```python
from build123d import *

# Parameters (mm, degrees)
SKETCH_1_R      = 2
SKETCH_1_R_2    = 2.08
SKETCH_1_R_3    = 8.75
SKETCH_1_R_4    = 2.2
EXTRUDE_2_DEPTH = 2


with BuildPart() as part:
    # 草图1 → 凸台-拉伸2 (new body)
    with BuildSketch(Plane.XY):
        with BuildLine():
            Line((41.5, 13.75), (41.5, 17))
            Line((41.5, 17), (37, 17))
            Line((37, 17), (37, 20))
            Line((37, 20), (30, 20))
            Line((30, 20), (30, 17))
            Line((30, 17), (25.488968202, 17))
            ThreePointArc((25.488968202, 17), (0, 27.55787632), (-25.488968202, 17))
            Line((-25.488968202, 17), (-30, 17))
            Line((-30, 17), (-30, 20))
            Line((-30, 20), (-37, 20))
            Line((-37, 20), (-37, 17))
            Line((-37, 17), (-41.5, 17))
            Line((-41.5, 17), (-41.5, 13.75))
            Line((-41.5, 13.75), (-44.5, 13.75))
            Line((-44.5, 13.75), (-44.5, 8.75))
            Line((-44.5, 8.75), (-41.5, 8.75))
            Line((-41.5, 8.75), (-41.5, 1.5))
            Line((-41.5, 1.5), (-39, 1.5))
            Line((-39, 1.5), (-39, 3))
            Line((-39, 3), (-36.4, 3))
            Line((-36.4, 3), (-36.4, 1.5))
            Line((-36.4, 1.5), (-33.4, 1.5))
            Line((-33.4, 1.5), (-33.4, -1.5))
            Line((-33.4, -1.5), (-36.4, -1.5))
            Line((-36.4, -1.5), (-36.4, -3))
            Line((-36.4, -3), (-39, -3))
            Line((-39, -3), (-39, -1.5))
            Line((-39, -1.5), (-41.5, -1.5))
            Line((-41.5, -1.5), (-41.5, -8.75))
            Line((-41.5, -8.75), (-44.5, -8.75))
            Line((-44.5, -8.75), (-44.5, -13.75))
            Line((-44.5, -13.75), (-41.5, -13.75))
            Line((-41.5, -13.75), (-41.5, -17))
            Line((-41.5, -17), (-37, -17))
            Line((-37, -17), (-37, -20))
            Line((-37, -20), (-30, -20))
            Line((-30, -20), (-30, -17))
            Line((-30, -17), (-25.488968202, -17))
            Line((-25.488968202, -17), (-4, -74.55787632))
            ThreePointArc((-4, -74.55787632), (0, -78.55787632), (4, -74.55787632))
            Line((4, -74.55787632), (25.488968202, -17))
            Line((25.488968202, -17), (30, -17))
            Line((30, -17), (30, -20))
            Line((30, -20), (37, -20))
            Line((37, -20), (37, -17))
            Line((37, -17), (41.5, -17))
            Line((41.5, -17), (41.5, -13.75))
            Line((41.5, -13.75), (44.5, -13.75))
            Line((44.5, -13.75), (44.5, -8.75))
            Line((44.5, -8.75), (41.5, -8.75))
            Line((41.5, -8.75), (41.5, -1.5))
            Line((41.5, -1.5), (39, -1.5))
            Line((39, -1.5), (39, -3))
            Line((39, -3), (36.4, -3))
            Line((36.4, -3), (36.4, -1.5))
            Line((36.4, -1.5), (33.4, -1.5))
            Line((33.4, -1.5), (33.4, 1.5))
            Line((33.4, 1.5), (36.4, 1.5))
            Line((36.4, 1.5), (36.4, 3))
            Line((36.4, 3), (39, 3))
            Line((39, 3), (39, 1.5))
            Line((39, 1.5), (41.5, 1.5))
            Line((41.5, 1.5), (41.5, 8.75))
            Line((41.5, 8.75), (44.5, 8.75))
            Line((44.5, 8.75), (44.5, 13.75))
            Line((44.5, 13.75), (41.5, 13.75))
        make_face()
        with Locations((0, -15)):
            Circle(SKETCH_1_R, mode=Mode.SUBTRACT)
        with Locations((-12.990381057, -7.5)):
            Circle(SKETCH_1_R, mode=Mode.SUBTRACT)
        with Locations((-12.990381057, 7.5)):
            Circle(SKETCH_1_R, mode=Mode.SUBTRACT)
        with Locations((0, 15)):
            Circle(SKETCH_1_R, mode=Mode.SUBTRACT)
        with Locations((12.990381057, 7.5)):
            Circle(SKETCH_1_R, mode=Mode.SUBTRACT)
        with Locations((12.990381057, -7.5)):
            Circle(SKETCH_1_R, mode=Mode.SUBTRACT)
        with Locations((-13.53, 0)):
            Circle(SKETCH_1_R_2, mode=Mode.SUBTRACT)
        with Locations((6.765, 11.717323713)):
            Circle(SKETCH_1_R_2, mode=Mode.SUBTRACT)
        with Locations((6.765, -11.717323713)):
            Circle(SKETCH_1_R_2, mode=Mode.SUBTRACT)
        Circle(SKETCH_1_R_3, mode=Mode.SUBTRACT)
        with Locations((0, -74.55787632)):
            Circle(SKETCH_1_R_4, mode=Mode.SUBTRACT)
    extrude(amount=EXTRUDE_2_DEPTH)


solid = part.part
```
Source: CAD feature listing. Evaluate the final solid. Frame: model axes, mm. Give positions to 0.01 mm unless a question says otherwise; leave off trailing zeros. Write each loop counter-clockwise with the first axis right and the second up, starting at its lowest first coordinate (ties: lowest second). Pieces come first, ordered by that corner, then holes.
1. Section query A-A (x = 35). Return the cut outline in (y, z).
2. Section query D-D (y = 18.5). Return the cut outline in (x, z) (3 decimals), then the cut area to 3 significant figures.
3. Material intervals for line 1 along Y through (x, z) = (0, 0.6); line 2 along Y through (x, z) = (-38.5, 1.85); line 3 along X through (y, z) = (-3.5, 1.1), sorted ascending.
4. Section query C-C (x = -13.53). Return the cut outline in (y, z).
5. Pull-direction query (X, two-part tool) for faces 1 (the face through (-0.088, -78.557, 0.986)), 2 (the face through (-11.083, 8.101, 0.986)), 3 (the face through (-1, -13, 0)); classes: +X half, -X half, draft (parallel to the pull), parting line (faces both ways), or undercut.
6. Section query B-B (y = -15). Return the cut outline in (x, z), then the cut area to 3 significant figures.
7. First-contact query: pin 1 (0.6 mm diameter, centred on x = 43.5, z = 1, fed in from +Y); pin 2 (1 mm diameter, centred on x = -34, z = 1, fed in from +Y); pin 3 (0.6 mm diameter, centred on y = -18, z = 1.5, fed in from -X). Flat tips, straight axial feed; report the tip coordinate or a pass-through.
Output values:
1. outline: (-20, 0) - (-1.5, 0) - (-1.5, 2) - (-20, 2) - close; (1.5, 0) - (20, 0) - (20, 2) - (1.5, 2) - close
2. outline: (-37, 0) - (-30, 0) - (-30, 2) - (-37, 2) - close; (-23.895, 0) - (23.895, 0) - (23.895, 2) - (-23.895, 2) - close; (30, 0) - (37, 0) - (37, 2) - (30, 2) - close
2. area: 124 mm2
3. line 1: y = -78.56 to -76.76, -72.36 to -17, -13 to -8.75, 8.75 to 13, 17 to 27.56
3. line 2: y = -17 to -3, 3 to 17
3. line 3: x = -41.5 to -8.02, 8.02 to 41.5
4. outline: (-49.03, 0) - (-9.43, 0) - (-9.43, 2) - (-49.03, 2) - close; (-5.57, 0) - (-2.08, 0) - (-2.08, 2) - (-5.57, 2) - close; (2.08, 0) - (5.57, 0) - (5.57, 2) - (2.08, 2) - close; (9.43, 0) - (24.92, 0) - (24.92, 2) - (9.43, 2) - close
5. face 1: parting line
5. face 2: undercut
5. face 3: draft
6. outline: (-41.5, 0) - (-2, 0) - (-2, 2) - (-41.5, 2) - close; (2, 0) - (41.5, 0) - (41.5, 2) - (2, 2) - close
6. area: 158 mm2
7. pin 1: stops at y = 13.75
7. pin 2: stops at y = 20
7. pin 3: stops at x = -37
